For this review, use the dimensioned drawing (mm, ordinates from the lowest corner) and the shaded views. A direction names the side the tool comes from. Coordinates: 2 decimals unless noted, no trailing zeros. Loops run counter-clockwise (first coordinate to the right, second up) from the corner with the lowest first, then second, coordinate; pieces in that order, holes last.
1. Take a section at A-A, the plane x = 61.5. State the section outline as (y, z) points, then the cut area to 3 significant figures.
2. Machinability: for the marked faces 1, 2 and 3, which of the approach directions +Z, -Z, +X, -X, +Y, -Y give a long, thin tool a straight path to every point of the face, cutting with its end or side? Answer none if there is none.
3. Take a section at D-D, the plane x = 37. State the section outline as (y, z) points, then the cut area to 3 significant figures.
4. Take a section at B-B, the plane z = 58.22. State the section outline as (x, y) points, then the cut area to 3 significant figures.
5. Take a section at C-C, the plane y = 1. State the section outline as (x, z) points.
6. Clearance check with flat-ended pins moving along their axes: P1, Ø1.7, axis at y = 7, z = 2.5, coming from the -X side; P2, Ø4.5, axis at y = 8.5, z = 3, coming from the +X side; P3, Ø1, axis at x = 56, z = 46, coming from the -Y side; P4, Ø2, axis at x = 3.5, z = 9.22, coming from the +Y side. State where each tip first meets the part, or that it passes through.
7. To check wall thickness, follow probe 1 along Z at (x, y) = (61.5, 4.5); probe 2 along X at (y, z) = (4.25, 9.22); probe 3 along X at (y, z) = (1.5, 10). State the ranges of each line that lie inside material, in increasing order.
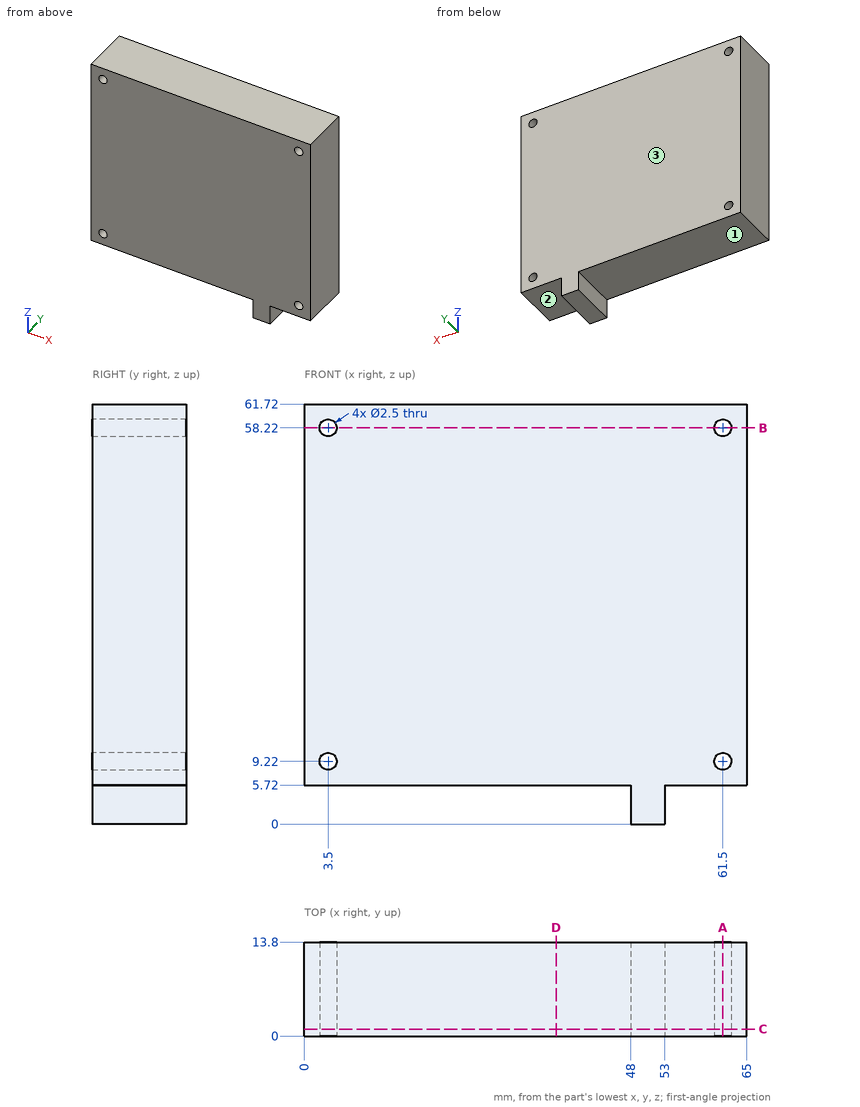
Results list:
1. outline: (0, 5.72) - (13.8, 5.72) - (13.8, 7.97) - (0, 7.97) - close; (0, 10.47) - (13.8, 10.47) - (13.8, 56.97) - (0, 56.97) - close; (0, 59.47) - (13.8, 59.47) - (13.8, 61.72) - (0, 61.72) - close
1. area: 704 mm2
2. face 1: -Z, -X, +Y, -Y
2. face 2: -Z, +X, +Y, -Y
2. face 3: +Z, -Z, +X, -X, +Y
3. outline: (0, 5.72) - (13.8, 5.72) - (13.8, 61.72) - (0, 61.72) - close
3. area: 773 mm2
4. outline: (0, 0) - (2.25, 0) - (2.25, 13.8) - (0, 13.8) - close; (4.75, 0) - (60.25, 0) - (60.25, 13.8) - (4.75, 13.8) - close; (62.75, 0) - (65, 0) - (65, 13.8) - (62.75, 13.8) - close
4. area: 828 mm2
5. outline: (0, 5.72) - (48, 5.72) - (48, 0) - (53, 0) - (53, 5.72) - (65, 5.72) - (65, 61.72) - (0, 61.72) - close; hole circle Ø2.5 at (3.5, 9.22); hole circle Ø2.5 at (3.5, 58.22); hole circle Ø2.5 at (61.5, 9.22); hole circle Ø2.5 at (61.5, 58.22)
6. P1: stops at x = 48
6. P2: stops at x = 53
6. P3: stops at y = 0
6. P4: passes through
7. probe 1: z = 5.72 to 7.97, 10.47 to 56.97, 59.47 to 61.72
7. probe 2: x = 0 to 2.25, 4.75 to 60.25, 62.75 to 65
7. probe 3: x = 0 to 2.52, 4.48 to 60.52, 62.48 to 65
